Read the model definition and answer for the solid it produces. Units are mm, in the model's axes. A direction names the side the tool comes from. Round coordinates to 2 decimals unless told otherwise and drop trailing zeros. Write each loop counter-clockwise with the first axis right and the second up, starting at its lowest first coordinate (ties: lowest second). Pieces come first, ordered by that corner, then holes. Notation, with made-up numbers: (-32.5, -5.5) -> (1.5, -5.5) arc R24 cw to (1.5, 20.5) -> close; hole circle Ø1 at (-34.5, 20.5). An arc over 180 degrees is marked (long way). Return JSON: item names as keys, results as strings. Group by question number.
(1) For faces 1 (the cylindrical face through (5.425, 5.257, 565.975)), 2 (the flat face through (-5, 0, -9)), 3 (the flat face through (377.5, 104, 8)), determine the directions among +Z, -Z, +X, -X, +Y, -Y from which every point of the face is accessible in a straight line to the end or side of a thin tool.
(2) A cutting plane is placed at C-C on z = -436.5. Give the vertices of the cut face in (x, y), then the cut area to 4 significant figures.
(3) The mould has two halves that part along Z. Classify faces 4 (the flat face through (-377.5, 104, 8)), 5 (the flat face through (-5, 99, -565)), 6 (the flat face through (-387.5, 88, 27)), 7 (the flat face through (-5, 104, 555)): released by +Z, released by -Z, zero draft, split by the parting line, or undercut.
(4) Given pin 1 (6 mm diameter, centred on x = -2, z = 210, fed in from +Y); pin 2 (5 mm diameter, centred on x = 122, z = 80, fed in from -Y); pin 3 (4 mm diameter, centred on x = -164.5, y = 10.5, fed in from +Z), each flat-ended and moving along its own axis, determine where each tip first touches the part or whether it passes through.
(5) Straight lines are drawn through the part: line 1 (X direction, y = 24, z = -263); line 2 (Z direction, x = 353, y = 116); line 3 (Y direction, x = 230, z = 512.5). For each, find the intervals that lie inside material, in ascending order.
(6) A cutting plane is placed at B-B on x = -191.5. Give the vertices of the cut face in (y, z), then the cut area to 3 significant figures.
(7) A cutting plane is placed at A-A on y = 61.5. Give the vertices of the cut face in (x, z), then the cut area to 3 significant figures.
```python
from build123d import *

# Parameters (mm, degrees)
SKETCH1_W           = 775
SKETCH1_H           = 1130
BOSS_EXTRUDE1_DEPTH = 200
SHELL1_T            = -10
SKETCH4_R           = 20
BOSS_EXTRUDE3_DEPTH = 775
SKETCH5_R           = 17.5
CUT_EXTRUDE2_DEPTH  = 1280


with BuildPart() as part:
    # Sketch1 → Boss-Extrude1 (new body)
    with BuildSketch(Plane(origin=(0, 0, 0), x_dir=(1, 0, 0), z_dir=(0, 1, 0))):
        Rectangle(SKETCH1_W, SKETCH1_H)
    extrude(amount=BOSS_EXTRUDE1_DEPTH)

    # Shell1
    shell1_openings = [part.faces().sort_by_distance(p)[0] for p in [
        (0, 200, 0),
    ]]
    offset(amount=SHELL1_T, openings=shell1_openings, kind=Kind.INTERSECTION)

    # Sketch4 → Boss-Extrude3 (add)
    with BuildSketch(Plane(origin=(387.5, 0, 0), x_dir=(0, 0, -1), z_dir=(1, 0, 0))):
        with Locations((-582.66692, 0)):
            Circle(SKETCH4_R)
    extrude(amount=-BOSS_EXTRUDE3_DEPTH)

    # Sketch5 → Cut-Extrude2 (cut)
    with BuildSketch(Plane(origin=(387.5, 0, 0), x_dir=(0, 0, -1), z_dir=(1, 0, 0))):
        with Locations((-582.66692, 0)):
            Circle(SKETCH5_R)
    extrude(amount=-CUT_EXTRUDE2_DEPTH, mode=Mode.SUBTRACT)


solid = part.part
```
Checks:
{
 "1": {"face 1": "+X, -X", "face 2": "-Z, +X, -X, -Y", "face 3": "+Y"},
 "2": {"outline": "(-387.5, 0) -> (387.5, 0) -> (387.5, 200) -> (377.5, 200) -> (377.5, 10) -> (-377.5, 10) -> (-377.5, 200) -> (-387.5, 200) -> close", "area": "11,550 mm^2"},
 "3": {"face 4": "undercut", "face 5": "released by -Z", "face 6": "zero draft", "face 7": "undercut"},
 "4": {"pin 1": "stops at y = 10", "pin 2": "stops at y = 0", "pin 3": "stops at z = 600.77"},
 "5": {"line 1": "x = -387.5 to -377.5, 377.5 to 387.5", "line 2": "z = -565 to -555, 555 to 565", "line 3": "y = 0 to 10"},
 "6": {"outline": "(0, -565) -> (200, -565) -> (200, -555) -> (10, -555) -> (10, 555) -> (200, 555) -> (200, 565) -> (9.37, 565) arc R20 ccw (long way) to (0, 562.67) -> close; hole circle Ø35 at (0, 582.67)", "area": "15,400 mm^2"},
 "7": {"outline": "(-387.5, -565) -> (387.5, -565) -> (387.5, 565) -> (-387.5, 565) -> close; hole (-377.5, -555) -> (377.5, -555) -> (377.5, 555) -> (-377.5, 555) -> close", "area": "37,700 mm^2"}
}
